Autodesk Inventor part; units mm, degrees
ref_plane "YZ Plane" through (0, 0, 0) normal (1, 0, 0) x (0, 1, 0)
ref_plane "XZ Plane" through (0, 0, 0) normal (0, 1, 0) x (-1, 0, 0)
ref_plane "XY Plane" through (0, 0, 0) normal (0, 0, 1) x (1, 0, 0)
sketch "Sketch1" plane through (0, 0, 0) normal (0, 0, 1) x (1, 0, 0)
  line L0 (-20.5, 15) -> (20.5, 15)
  line L1 (20.5, 15) -> (20.5, -15)
  line L2 (20.5, -15) -> (-20.5, -15)
  line L3 (-20.5, -15) -> (-20.5, 15)
  line L4 (-20.5, 15) -> (20.5, -15) construction
  line L5 (20.5, 15) -> (-20.5, -15) construction
  circle A0 centre (0, 0) radius 11.35
  line L6 (16.5, 15) -> (16.5, -15)
  dimension "d0" = 41
  dimension "d1" = 30
  dimension "d2" = 22.7
  dimension "d4" = 4
extrude "Extrusion3" add sketch "Sketch1" along normal blind 10
sketch "Sketch3" plane through (0, 0, 0) normal (0, 0, -1) x (-1, 0, 0)
  circle A0 centre (0, 0) radius 11.35
  circle A1 centre (0, 0) radius 11.35
  circle A2 centre (0, 0) radius 8.5
  dimension "d18" = 17
extrude "Extrusion4" add sketch "Sketch3" against normal blind 3
sketch "Sketch4" plane through (-20.5, -15, 0) normal (0, -1, 0) x (1, 0, 0)
  line L0 (0, 0) -> (0, 10)
  line L1 (0, 0) -> (41, 0)
  line L2 (41, 0) -> (41, 20)
  line L3 (41, 20) -> (0, 20)
  line L4 (0, 20) -> (0, 0)
  point P0 (20.5, 0)
  dimension "d21" = 20
  dimension "d22" = 41
extrude "Extrusion5" add sketch "Sketch4" along normal blind 6
sketch "Sketch5" plane through (-20.5, -15, 20) normal (0, 0, 1) x (1, 0, 0)
  line L0 (0, 30) -> (0, 0)
  line L1 (0, 0) -> (41, 0)
  line L2 (41, 0) -> (41, -33.5)
  line L3 (41, -33.5) -> (0, -33.5)
  line L4 (0, -33.5) -> (0, 0)
  point P0 (20.5, 15)
  dimension "d25" = 33.5
  dimension "d69" = 41
extrude "Extrusion6" add sketch "Sketch5" along normal blind 6
sketch "Sketch13" plane through (20.5, 15, 10) normal (1, 0, 0) x (0, 0, -1)
  line L0 (-10, -63.5) -> (-16, -63.5)
  line L1 (-10, -63.5) -> (-10, -36)
  line L2 (-16, -63.5) -> (-10, -63.5)
  line L3 (-10, -63.5) -> (10, -36)
  line L4 (10, -36) -> (10, -30)
  line L5 (0, 0) -> (0, -30)
  line L6 (10, -30) -> (-16, -30)
  line L7 (-16, -30) -> (-16, -63.5)
  line L8 (-16, -30) -> (-16, -63.5)
  point P0 (10, -15)
  point P1 (-16, -56.5)
extrude "Extrusion10" add sketch "Sketch13" against normal blind 2
ref_plane "Work Plane1" through (0, 15, 0) normal (-1, 0, 0) x (0, 0, 1)
mirror "Mirror1" about plane through (0, 15, 0) normal (-1, 0, 0) of "Extrusion10"
fillet "Fillet2" radius 2 4 edges at (20.5, 15, 5) (-20.5, 15, 5) (0, 15, 10) (0, 15, 0)
sketch "Sketch15" plane through (-20.5, -15, 26) normal (0, 0, 1) x (1, 0, 0)
  arc A0 (13, -11.5) -> (7.5, -11.5) centre (10.25, -11.5) ccw
  line L0 (2, -33.5) -> (39, -33.5)
  line L1 (0, -2) -> (0, -31.5)
  arc A1 (7.5, -28.5) -> (13, -28.5) centre (10.25, -28.5) ccw
  line L2 (7.5, -11.5) -> (7.5, -28.5)
  line L3 (13, -11.5) -> (13, -28.5)
  line L4 (20.5, -33.5) -> (20.5, -2)
  arc A2 (33.5, -11.5) -> (28, -11.5) centre (30.75, -11.5) ccw
  arc A3 (28, -28.5) -> (33.5, -28.5) centre (30.75, -28.5) ccw
  line L5 (33.5, -11.5) -> (33.5, -28.5)
  line L6 (28, -11.5) -> (28, -28.5)
  point P0 (20.5, 15)
  dimension "d74" = 5.5
  dimension "d75" = 22
  dimension "d76" = 10.25
  dimension "d77" = 5.5
  dimension "d78" = 5
  dimension "d79" = 10.25
extrude "Extrusion11" cut sketch "Sketch15" against normal through all
properties part number "Estrutura - Rolamento Esquerdo"
For this review, take the finished solid that the model builds, in its own axes (mm). A direction names the side the tool comes from. Coordinates: 2 decimals unless noted, no trailing zeros. Order: outer loops, then holes, each group sorted by start corner. A loop starts at its lowest first (then second) coordinate and runs counter-clockwise, first axis right, second up. Notation, with made-up numbers: (-14.75, 48) -> (17.25, 48) arc R23 cw to (17.25, 66) -> close; hole circle Ø6 at (-13.75, 85). An arc over 180 degrees is marked (long way). Return JSON: item names as keys, results as strings.
1. We need section C-C on y = -40. Write out the cut boundary in (x, z), and give its area (3 significant figures).
Answer block:
{"outline": "(-20.5, 13.82) -> (-18.5, 13.82) -> (-18.5, 20) -> (-13, 20) -> (-13, 26) -> (-20.5, 26) -> close; (-7.5, 20) -> (7.5, 20) -> (7.5, 26) -> (-7.5, 26) -> close; (13, 20) -> (18.5, 20) -> (18.5, 13.82) -> (20.5, 13.82) -> (20.5, 26) -> (13, 26) -> close", "area": "205 mm²"}
2. We need section A-A on x = 0. Write out the cut boundary in (y, z).
Answer block:
{"outline": "(-48.5, 20) -> (-21, 20) -> (-21, 0) -> (-8.5, 0) -> (-8.5, 3) -> (-11.35, 3) -> (-11.35, 10) -> (-15, 10) -> (-15, 26) -> (-48.5, 26) -> close; (8.5, 0) -> (13, 0) arc R2 ccw to (15, 2) -> (15, 8) arc R2 ccw to (13, 10) -> (11.35, 10) -> (11.35, 3) -> (8.5, 3) -> close"}
3. For pin 1 Ø6 at (y, z) = (-5.5, 11) entering from -X; pin 2 Ø1.5 at (x, y) = (11, -25) entering from +Z; pin 3 Ø7 at (x, y) = (4.5, 3) entering from +Z; pin 4 Ø5 at (x, z) = (16, 20) entering from +Y, all flat-tipped, find the tip position at first contact; note any pin that passes through.
Answer block:
{"pin 1": "x = -20.5", "pin 2": "through", "pin 3": "z = 3", "pin 4": "y = -15"}
4. For line 1 (X direction, y = -29, z = 11); line 2 (Y direction, x = 0, z = 7); line 3 (Z direction, x = 11, y = 7.5), list the stretches that pass through material, from the lowest coordinate up. Write a range as from..to.
Answer block:
{"line 1": "-20.5..-18.5, 18.5..20.5", "line 2": "-21..-11.35, 11.35..15", "line 3": "0..10"}
5. Machinability: for faces 1 (the flat face through (0, -48.5, 23)), 2 (the flat face through (0, -35, 20)), 3 (the cylindrical face through (-10.19, -23.75, 23.04)), 4 (the flat face through (0, -15, 18)), 5 (the flat face through (0, -32, 26)), which of the approach directions +Z, -Z, +X, -X, +Y, -Y give a long, thin tool a straight path to every point of the face, cutting with its end or side? Answer none if there is none.
Answer block:
{"face 1": "+Z, -Z, +X, -X, -Y", "face 2": "-Z, -Y", "face 3": "+Z, -Z", "face 4": "+Z, +X, -X, +Y", "face 5": "+Z, +X, -X, +Y, -Y"}
6. We need section D-D on y = 9.5. Write out the cut boundary in (x, z).
Answer block:
{"outline": "(-20.5, 0) -> (20.5, 0) -> (20.5, 10) -> (6.21, 10) -> (6.21, 3) -> (-6.21, 3) -> (-6.21, 10) -> (-20.5, 10) -> close"}
7. We need section B-B on z = 21. Write out the cut boundary in (x, y), and give its area (3 significant figures).
Answer block:
{"outline": "(-20.5, -48.5) -> (20.5, -48.5) -> (20.5, -15) -> (-20.5, -15) -> close; hole (-13, -43.5) arc R2.75 ccw to (-7.5, -43.5) -> (-7.5, -26.5) arc R2.75 ccw to (-13, -26.5) -> close; hole (7.5, -43.5) arc R2.75 ccw to (13, -43.5) -> (13, -26.5) arc R2.75 ccw to (7.5, -26.5) -> close", "area": "1,140 mm²"}
8. The part is to be moulded in two halves that separate along X. For faces 6 (the flat face through (-20.5, -18, 13)), 7 (the flat face through (-9.4, -7, 10)), 8 (the flat face through (-13, -35, 23)), say which applies: +X half, -X half, draft (parallel to the pull), parting line (faces both ways), or undercut.
Answer block:
{"face 6": "-X half", "face 7": "draft", "face 8": "undercut"}
